Can you work these out from the drawing? Everything is in mm from the part's minimum corner. Round coordinates to 2 decimals unless told otherwise and drop trailing zeros. Order: outer loops, then holes, each group sorted by start corner. A loop starts at its lowest first (then second) coordinate and runs counter-clockwise, first axis right, second up. Notation, with made-up numbers: M -2.75,-19.75 L 6.25,-19.75 A33 ccw 6.25,16.25 Z; hole C -33.75,-38 d1. An arc over 180 degrees is marked long. Write each question's results on one line, items separated by ' | '. Start each with the question number.
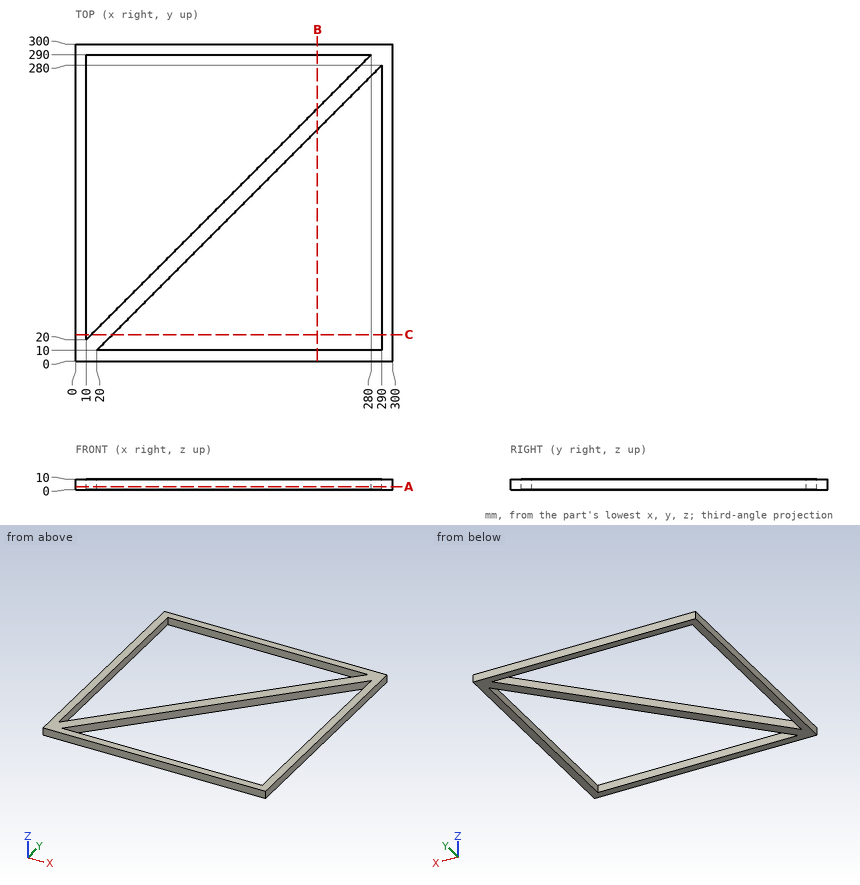
(1) I want a section at C-C on y = 25. Write out the boundary of the cut face in (x, z).
(2) Please list where these lines run through material, in increasing order: line 1 (Y direction, x = 76, z = 2); line 2 (Y direction, x = 39.5, z = 2.75); line 3 (X direction, y = 61, z = 1.25).
(3) I want a section at B-B on x = 229. Write out the boundary of the cut face in (y, z), and give its area (3 significant figures).
(4) I want a section at A-A on z = 2.75. Write out the boundary of the cut face in (x, y).
Solutions:
1) outline: M 0,0 L 10,0 L 10,10 L 0,10 Z; M 15,0 L 35,0 L 35,10 L 15,10 Z; M 290,0 L 300,0 L 300,10 L 290,10 Z
2) line 1: 0 to 10, 66 to 86, 290 to 300 | line 2: 0 to 10, 29.5 to 49.5, 290 to 300 | line 3: 0 to 10, 51 to 71, 290 to 300
3) outline: M 0,0 L 10,0 L 10,10 L 0,10 Z; M 219,0 L 239,0 L 239,10 L 219,10 Z; M 290,0 L 300,0 L 300,10 L 290,10 Z | area: 400 mm^2
4) outline: M 0,0 L 300,0 L 300,300 L 0,300 Z; hole M 10,20 L 280,290 L 10,290 Z; hole M 20,10 L 290,10 L 290,280 Z
